Drawing for the job (mm, zero at the part's lowest x, y, z). A direction names the side the tool comes from. Coordinates: 2 decimals unless noted, no trailing zeros. Loops run counter-clockwise (first coordinate to the right, second up) from the corner with the lowest first, then second, coordinate; pieces in that order, holes last. Notation, with made-up numbers: (62.5, 5.5) -> (113.5, 5.5) arc R20 cw to (113.5, 10.5) -> close; hole circle Ø4 at (86.5, 52.5). An arc over 180 degrees is marked (long way). Write item = value, one per line. Start each with the question number.
(1) Band-saw the part on C-C (x = 11). Write the cut outline in (y, z).
(2) Band-saw the part on D-D (z = 5). Write the cut outline in (x, y).
(3) Tool access for the marked faces 1, 2 and 3: list every direction of +Z, -Z, +X, -X, +Y, -Y with a clear straight run to the whole face (end or side of a thin tool).
(4) Flat gauge pins, fed straight in: P1, Ø0.5, axis at y = 4.5, z = 6.5, coming from the +X side; P2, Ø0.5, axis at y = 4, z = 15.5, coming from the +X side; P3, Ø1.8, axis at y = 5, z = 6, coming from the -X side. Where does each tip first touch, or does it go through?
(5) Pull direction X, two halves, no side cores. Call the marked faces 4, 5, 6 and 7: +X half, -X half, draft (parallel to the pull), parting line (faces both ways), or undercut.
(6) Drill centre lines: line 1 (Z direction, x = 11, y = 4.75); line 2 (Z direction, x = 9.75, y = 6.5); line 3 (Y direction, x = 18.5, z = 12.5). Where is each one in solid material? Low to high. Write a range as from..to.
(7) Band-saw the part on A-A (y = 4). Write the cut outline in (x, z).
(8) Band-saw the part on B-B (z = 11). Write the cut outline in (x, y), and give its area (3 significant figures).
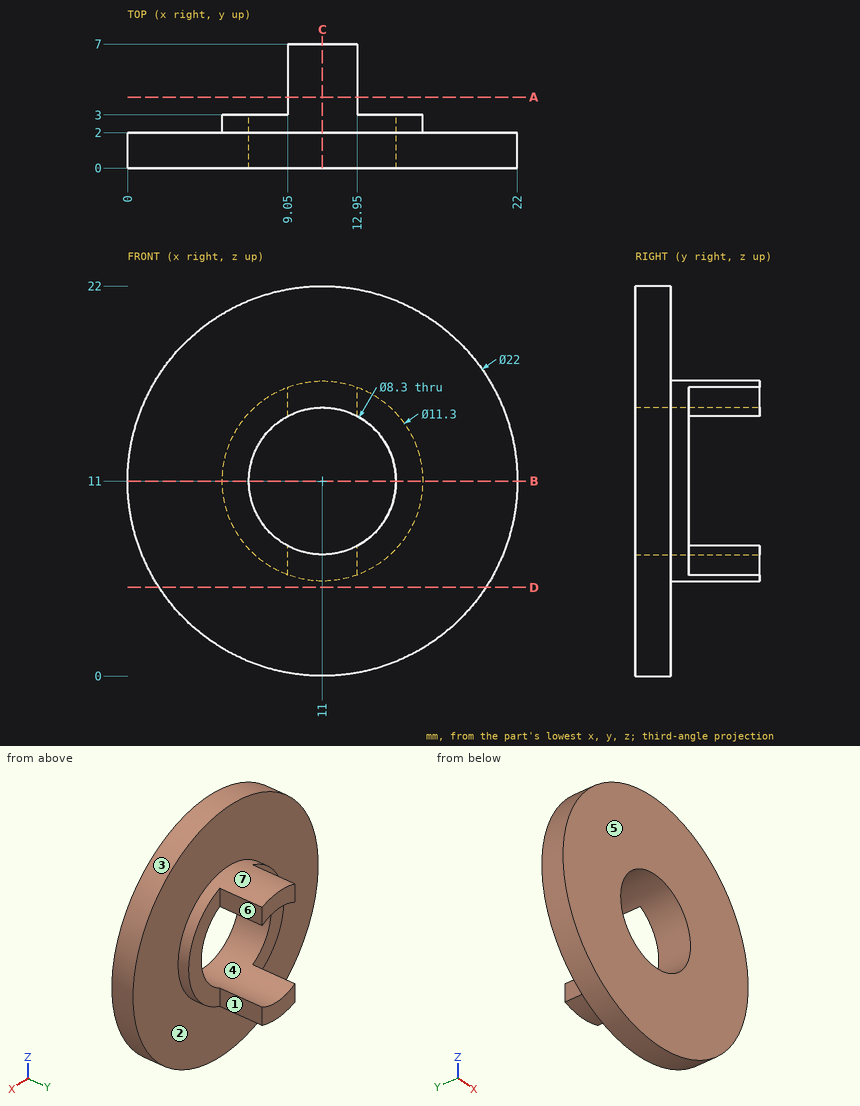
Findings below:
q1.outline = (0, 0) -> (2, 0) -> (2, 5.35) -> (7, 5.35) -> (7, 6.85) -> (0, 6.85) -> close; (0, 15.15) -> (7, 15.15) -> (7, 16.65) -> (2, 16.65) -> (2, 22) -> (0, 22) -> close
q2.outline = (1.78, 0) -> (20.22, 0) -> (20.22, 2) -> (1.78, 2) -> close
q3.face_1 = +Z, -Z, +X, +Y
q3.face_2 = +Y
q3.face_3 = +Y, -Y
q4.P1 = 12.95
q4.P2 = 12.95
q4.P3 = 9.05
q5.face_4 = undercut
q5.face_5 = draft
q5.face_6 = +X half
q5.face_7 = parting line
q6.line_1 = 5.35..6.85, 15.15..16.65
q6.line_2 = 5.49..7.04, 14.96..16.51
q6.line_3 = 0..2
q7.outline = (9.05, 5.7) arc R5.65 ccw to (12.95, 5.7) -> (12.95, 7.34) arc R4.15 cw to (9.05, 7.34) -> close; (9.05, 14.66) arc R4.15 cw to (12.95, 14.66) -> (12.95, 16.3) arc R5.65 ccw to (9.05, 16.3) -> close
q8.outline = (0, 0) -> (6.85, 0) -> (6.85, 3) -> (5.35, 3) -> (5.35, 2) -> (0, 2) -> close; (15.15, 0) -> (22, 0) -> (22, 2) -> (16.65, 2) -> (16.65, 3) -> (15.15, 3) -> close
q8.area = 30.4 mm²
